```python
from build123d import *

# Parameters (mm, degrees)
SKETCH1_R                  = 40
SKETCH1_R_2                = 10
BOSS_EXTRUDE1_DEPTH        = 10
M12X1_5_TAPPED_HOLE1_D     = 10.5
CIRPATTERN1_COUNT          = 6
SKETCH5_R                  = 17.5
SKETCH5_R_2                = 10
BOSS_EXTRUDE2_DEPTH        = 10
M6X1_0_TAPPED_HOLE1_REACH  = 74.844
M6X1_0_TAPPED_HOLE1_BORE_R = 2.5
FILLET1_R                  = 1


with BuildPart() as part:
    # Sketch1 → Boss-Extrude1 (new body)
    with BuildSketch(Plane.XY):
        Circle(SKETCH1_R)
        Circle(SKETCH1_R_2, mode=Mode.SUBTRACT)
    extrude(amount=BOSS_EXTRUDE1_DEPTH)

    # M12x1.5 Tapped Hole1 (through all)
    with Locations(Plane.XY.offset(10)):
        with Locations((0, 25)):
            m12x1_5_tapped_hole1 = Hole(M12X1_5_TAPPED_HOLE1_D / 2)

    # CirPattern1: M12x1.5 Tapped Hole1 ×6 about axis
    cirpattern1_axis = Axis((0, 0, 0), (0, 0, 1))
    for i in range(1, CIRPATTERN1_COUNT):
        add(m12x1_5_tapped_hole1.rotate(cirpattern1_axis, i * 360 / CIRPATTERN1_COUNT), mode=Mode.SUBTRACT)

    # Sketch5 → Boss-Extrude2 (add)
    with BuildSketch(Plane.XY.offset(10)):
        Circle(SKETCH5_R)
        Circle(SKETCH5_R_2, mode=Mode.SUBTRACT)
    extrude(amount=BOSS_EXTRUDE2_DEPTH)

    # M6x1.0 Tapped Hole1 bore → M6x1.0 Tapped Hole1 (cut, up to next)
    with BuildSketch(Plane(origin=(0, 17.5, 0), x_dir=(1, 0, 0), z_dir=(0, 1, 0)), mode=Mode.PRIVATE) as m6x1_0_tapped_hole1_sk1:
        with Locations((0, -15)):
            Circle(M6X1_0_TAPPED_HOLE1_BORE_R)
    m6x1_0_tapped_hole1_tool1 = extrude(m6x1_0_tapped_hole1_sk1.sketch, amount=-M6X1_0_TAPPED_HOLE1_REACH, mode=Mode.PRIVATE) & part.part
    add(m6x1_0_tapped_hole1_tool1.solids().sort_by_distance((0, 17.5, 15))[0], mode=Mode.SUBTRACT)

    # Fillet1
    fillet1_edges = [part.edges().sort_by_distance(p)[0] for p in [
        (-40, 0, 0),
        (-17.5, 0, 10),
        (-17.5, 0, 20),
        (-40, 0, 10),
    ]]
    fillet(fillet1_edges, radius=FILLET1_R)


solid = part.part
```
Check sheet for the modelled part. Datum: model origin and axes. Units: mm. A direction names the side the tool comes from. Round coordinates to 2 decimals unless told otherwise and drop trailing zeros. Loops run counter-clockwise (first coordinate to the right, second up) from the corner with the lowest first, then second, coordinate; pieces in that order, holes last. Notation, with made-up numbers: (71.25, -9.5) - (116.25, -9.5) arc R29 cw to (116.25, 18.5) - close; hole circle Ø7 at (13.5, -31.75). An arc over 180 degrees is marked (long way). Write item = value, one per line. Start each with the question number.
Q1. Section check B-B (y = 0). Record the boundary of the cut face in (x, z), plus the area to 3 significant figures.
Q2. Release check for a two-part mould opening along Z. For faces 1 (the face through (-0.54, 13.64, 17.44)), 2 (the face through (8, -8, 0)), 3 (the face through (-1.138, -19.875, 4.93)) record: pulls with the +Z half, pulls with the -Z half, needs draft (parallel to the pull), parting line crosses it, or undercut.
Q3. Depth check by flat-ended pin: P1, Ø8, axis at y = -16, z = 5, coming from the -X side; P2, Ø8.5, axis at x = -21.65, y = 12.5, coming from the +Z side; P3, Ø12, axis at x = -2.5, z = 2.5, coming from the -Y side; P4, Ø6, axis at x = -3, z = 11.5, coming from the +Y side. Enter the tip coordinate at first touch or a pass-through.
Q4. Thickness scan on L1, parallel to Y at x = 0, z = 3.5; L2, parallel to Z at x = 0, y = 16; L3, parallel to Z at x = -26.5, y = 3.5. Record the ranges inside material, lowest first.
Q5. Section check D-D (z = 5.25). Record the boundary of the cut face in (x, y).
Q6. Section check A-A (x = 0). Count the separate pieces of the cut face and the enclosed holes in it, plus the area to 3 significant figures.
Q7. Access from +Z, -Z, +X, -X, +Y, -Y to the whole of each face (thin tool, end or side, straight path). Record for faces 4 (the face through (0, -11, 20)), 5 (the face through (8, -17, 10)).
Derived:
q1.outline = (-40, 1) arc R1 ccw to (-39, 0) - (-10, 0) - (-10, 20) - (-16.5, 20) arc R1 ccw to (-17.5, 19) - (-17.5, 11) arc R1 cw to (-18.5, 10) - (-39, 10) arc R1 ccw to (-40, 9) - close; (10, 0) - (39, 0) arc R1 ccw to (40, 1) - (40, 9) arc R1 ccw to (39, 10) - (18.5, 10) arc R1 cw to (17.5, 11) - (17.5, 19) arc R1 ccw to (16.5, 20) - (10, 20) - close
q1.area = 749 mm^2
q2.face_1 = undercut
q2.face_2 = pulls with the -Z half
q2.face_3 = needs draft
q3.P1 = -38.16
q3.P2 = through
q3.P3 = -40
q3.P4 = 39.98
q4.L1 = -40 to -30.25, -19.75 to -10, 10 to 19.75, 30.25 to 40
q4.L2 = 0 to 12.5, 17.5 to 20
q4.L3 = 0 to 10
q5.outline = circle Ø80 at (0, 0); hole circle Ø10.5 at (-21.65, -12.5); hole circle Ø10.5 at (-21.65, 12.5); hole circle Ø20 at (0, 0); hole circle Ø10.5 at (0, -25); hole circle Ø10.5 at (0, 25); hole circle Ø10.5 at (21.65, -12.5); hole circle Ø10.5 at (21.65, 12.5)
q6.separate_pieces = 5
q6.enclosed_holes = 0
q6.area = 502 mm^2
q7.face_4 = +Z, +X, -X, +Y, -Y
q7.face_5 = +Z
